Can you work these out from the drawing? Everything is in mm from the part's minimum corner. A direction names the side the tool comes from. Give positions to 0.01 mm unless a question says otherwise; leave off trailing zeros. Write each loop counter-clockwise with the first axis right and the second up, starting at its lowest first coordinate (ties: lowest second). Pieces come first, ordered by that corner, then holes. Notation, with made-up numbers: (-12, 7.25) - (35, 7.25) arc R11 cw to (35, 18.25) - close; hole circle Ø5 at (25, 16). An arc over 180 degrees is marked (long way). Use a Markdown table: item, result. Add a question column.
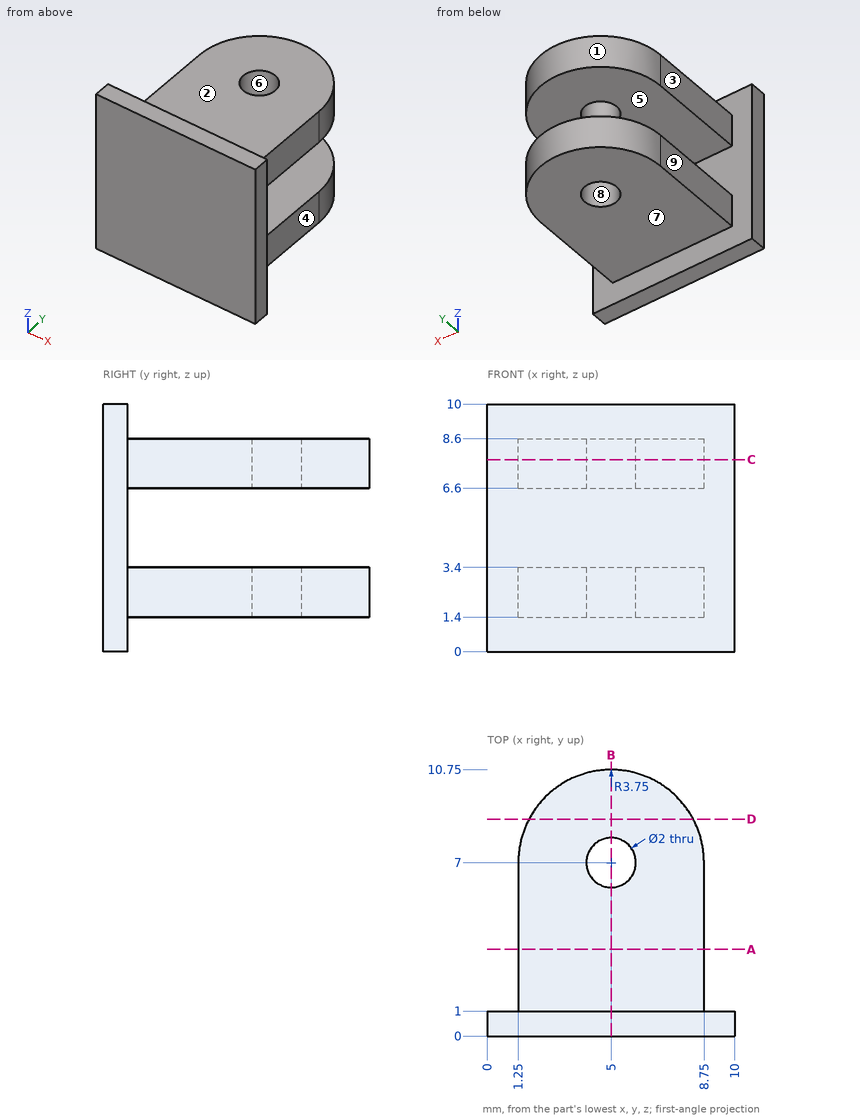
Q1. Suppose I cut it at C-C (z = 7.75). Please give me the cut outline in (x, y), and give its area (3 significant figures).
Q2. Suppose I cut it at B-B (x = 5). Please give me the cut outline in (y, z).
Q3. On a 3-axis mill with a long thin cutter (end or side, diameter ignored), from which of +Z, -Z, +X, -X, +Y, -Y can I reach the whole of each face in a straight line? I mean the marked faces 1, 2, 3, 4 and 5. Say none if no direction works.
Q4. If we mould it in two halves opening along X, with no side actions, what happens to the marked faces 6, 7, 8 and 9? For each: released by +X, released by -X, zero draft, split by the parting line, or undercut.
Q5. Suppose I cut it at D-D (y = 8.75). Please give me the cut outline in (x, z), and give its area (3 significant figures).
Q6. Suppose I cut it at A-A (y = 3.5). Please give me the cut outline in (x, z).
Q7. I'm going to push flat-ended pins straight in: P1, Ø5, axis at x = 5.5, y = 6, coming from the -Z side; P2, Ø5, axis at y = 9.5, z = 2.5, coming from the +X side; P3, Ø1.6, axis at y = 5, z = 7.5, coming from the -X side; P4, Ø3, axis at x = 3, z = 2, coming from the -Y side. Where does each tip first touch, or does it pass through?
Q8. If I drill on probe 1 along Z at (x, y) = (4.25, 3); probe 2 along Y at (x, z) = (5, 7.55); probe 3 along Y at (x, z) = (7.25, 7), over which ranges is the centre line in solid material (lowest first)? Write a range as [from, to].
Derived:
| question | item | result |
|---|---|---|
| 1 | outline | (0, 0) - (10, 0) - (10, 1) - (8.75, 1) - (8.75, 7) arc R3.75 ccw to (1.25, 7) - (1.25, 1) - (0, 1) - close; hole circle Ø2 at (5, 7) |
| 1 | area | 73.9 mm² |
| 2 | outline | (0, 0) - (1, 0) - (1, 1.4) - (6, 1.4) - (6, 3.4) - (1, 3.4) - (1, 6.6) - (6, 6.6) - (6, 8.6) - (1, 8.6) - (1, 10) - (0, 10) - close; (8, 1.4) - (10.75, 1.4) - (10.75, 3.4) - (8, 3.4) - close; (8, 6.6) - (10.75, 6.6) - (10.75, 8.6) - (8, 8.6) - close |
| 3 | face 1 | +Z, -Z, +Y |
| 3 | face 2 | +Z, +X, -X, +Y |
| 3 | face 3 | +Z, -Z, -X, +Y |
| 3 | face 4 | +Z, -Z, +X, +Y |
| 3 | face 5 | +X, -X, +Y |
| 4 | face 6 | undercut |
| 4 | face 7 | zero draft |
| 4 | face 8 | undercut |
| 4 | face 9 | released by -X |
| 5 | outline | (1.68, 1.4) - (8.32, 1.4) - (8.32, 3.4) - (1.68, 3.4) - close; (1.68, 6.6) - (8.32, 6.6) - (8.32, 8.6) - (1.68, 8.6) - close |
| 5 | area | 26.5 mm² |
| 6 | outline | (1.25, 1.4) - (8.75, 1.4) - (8.75, 3.4) - (1.25, 3.4) - close; (1.25, 6.6) - (8.75, 6.6) - (8.75, 8.6) - (1.25, 8.6) - close |
| 7 | P1 | z = 1.4 |
| 7 | P2 | x = 8.75 |
| 7 | P3 | x = 1.25 |
| 7 | P4 | y = 0 |
| 8 | probe 1 | [1.4, 3.4], [6.6, 8.6] |
| 8 | probe 2 | [0, 6], [8, 10.75] |
| 8 | probe 3 | [0, 10] |
